Autodesk Inventor part; units mm, degrees
ref_plane "YZ Plane" through (0, 0, 0) normal (1, 0, 0) x (0, 1, 0)
ref_plane "XZ Plane" through (0, 0, 0) normal (0, 1, 0) x (-1, 0, 0)
ref_plane "XY Plane" through (0, 0, 0) normal (0, 0, 1) x (1, 0, 0)
sketch "Sketch1" plane through (0, 0, 0) normal (1, 0, 0) x (0, 1, 0)
  line L0 (0, 0) -> (10, 0)
  line L1 (10, 0) -> (10, 20)
  line L2 (10, 20) -> (5, 40)
  line L3 (5, 40) -> (0, 40)
  line L4 (0, 40) -> (0, 0)
  dimension "d0" = 10
  dimension "d1" = 5
  dimension "d2" = 20
  dimension "d3" = 20
extrude "Extrusion1" add sketch "Sketch1" along normal mid plane 20
sketch "Sketch2" plane through (-10, 0, 40) normal (0, 0, 1) x (1, 0, 0)
  line L0 (7.1, -1) -> (12.9, -1)
  line L1 (12.9, -1) -> (12.9, 0)
  line L2 (12.9, 0) -> (7.1, 0)
  line L3 (7.1, 0) -> (7.1, -1)
  line L4 (7.1, -1) -> (12.9, 0) construction
  line L5 (12.9, -1) -> (7.1, 0) construction
  line L6 (0, 0) -> (20, 0)
  point P0 (10, 0)
  point P1 (10, -0.5)
  point P2 (10, 0)
  dimension "d6" = 5.8
  dimension "d7" = 1
extrude "Extrusion2" add sketch "Sketch2" against normal up to surface (40 mm away)
sketch "Sketch5" plane through (10, 0, 0) normal (1, 0, 0) x (0, 0, -1)
  line L0 (-12.875, 11) -> (-7.125, 11)
  line L1 (-7.125, 11) -> (-7.125, 10)
  line L2 (-7.125, 10) -> (-12.875, 10)
  line L3 (-12.875, 10) -> (-12.875, 11)
  line L4 (-12.875, 11) -> (-7.125, 10) construction
  line L5 (-7.125, 11) -> (-12.875, 10) construction
  line L6 (0, 10) -> (-20, 10)
  point P0 (0, 0)
  point P1 (-10, 10.5)
  point P2 (-10, 10)
  dimension "d24" = 5.75
  dimension "d25" = 1
extrude "Extrusion3" add sketch "Sketch5" against normal up to surface (20 mm away)
chamfer "Chamfer1" distance 1 angle 45 1 edges at (0, 11, 7.125)
sketch "Sketch3" plane through (-10, 10, 20) normal (0, 1, 0) x (1, 0, 0)
  line L0 (0, -20) -> (20, -20)
  line L1 (20, 0) -> (20, -20)
  line L2 (0, 0) -> (20, 0)
  line L3 (0, -20) -> (0, 0)
  point P0 (10, 20)
  point P1 (10, -10)
  point P2 (10, 0)
  point P3 (0, -10)
hole "Hole1" at (0, 10, 30) direction (0, -1, 0) diameter 5.5 end through all counterbore diameter 10 counterbore depth 5
sketch "Sketch4" plane through (-2.9, -1, 40) normal (0, -1, 0) x (1, 0, 0)
  line L0 (-7.1, -20) -> (12.9, -20)
  line L1 (12.9, -40) -> (12.9, -32.875)
  line L2 (12.9, -40) -> (-7.1, -40)
  line L3 (-7.1, -20) -> (-7.1, -27.125)
  line L4 (-7.1, -32.875) -> (12.9, -32.875)
  line L5 (-7.1, -32.875) -> (-7.1, -40)
  line L6 (12.9, -27.125) -> (-7.1, -27.125)
  line L7 (12.9, -27.125) -> (12.9, -20)
  line L8 (-7.1, -32.875) -> (12.9, -32.875)
  line L9 (2.9, -32.875) -> (2.9, -27.125) construction
  line L10 (12.9, -27.125) -> (-7.1, -27.125)
  point P0 (2.9, -40)
  point P1 (2.9, -30)
  point P2 (-7.1, -23.5625)
  point P3 (2.9, -20)
  point P4 (2.9, -30)
hole "Hole2" at (0, -1, 10) direction (0, 1, 0) diameter 5.5 end through all counterbore diameter 10 counterbore depth 7.25
fillet "Fillet1" radius 1 5 edges at (0, 5, 40) (-10, 7.5, 30) (10, 7.5, 30) (10, 2.5, 40) (-10, 2.5, 40)
properties part number "Y-Axis_Extursion_Mount_LM3041" material "ABS Plastic"
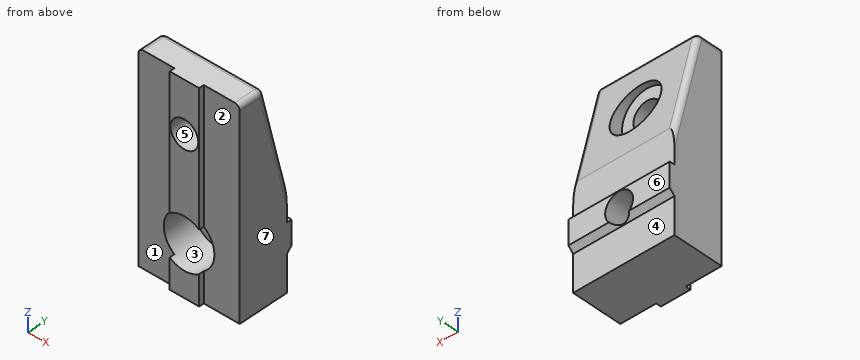
Geometry check sheet. Reference: the model listing, model coordinates, mm. Face numbers are marked on the shaded views. A direction names the side the tool comes from. Round coordinates to 2 decimals unless told otherwise and drop trailing zeros. Write each loop counter-clockwise with the first axis right and the second up, starting at its lowest first coordinate (ties: lowest second). Pieces come first, ordered by that corner, then holes. Notation, with made-up numbers: (-8, 57.25) - (46, 57.25) arc R13 ccw to (46, 79.25) - close; hole circle Ø11 at (12.25, -11). An arc over 180 degrees is marked (long way). Write each question's results on one line, items separated by ' | '.
(1) Depth check by flat-ended pin: pin 1 Ø8 at (x, z) = (0, 30) entering from +Y; pin 2 Ø5.5 at (x, z) = (-0.5, 16.5) entering from +Y; pin 3 Ø8 at (x, z) = (0, 10) entering from -Y. Enter the tip coordinate at first touch or a pass-through.
Computed:
pin 1: stops at y = 5 | pin 2: stops at y = 10 | pin 3: stops at y = 6.25
(2) Sectioned sample at B-B, the plane z = 10. Enter the section's corners in (x, y).
Computed:
outline: (-10, 0) - (-5, 0) - (-5, 6.25) - (-2.75, 6.25) - (-2.75, 11) - (-10, 11) - close; (2.75, 6.25) - (5, 6.25) - (5, 0) - (10, 0) - (10, 11) - (2.75, 11) - close
(3) Thickness scan on probe 1 along Z at (x, y) = (0, 2.25); probe 2 along X at (y, z) = (4.75, 10); probe 3 along X at (y, z) = (2.95, 30). Record the ranges inside material, lowest first. Write a range as from..to.
Computed:
probe 1: z = 0..5, 15..27.25, 32.75..40 | probe 2: x = -10..-5, 5..10 | probe 3: x = -10..-2.75, 2.75..10
(4) Sectioned sample at C-C, the plane x = 0. Count the separate pieces of the cut face and the enclosed holes in it, plus the area to 3 significant figures.
Computed:
separate pieces: 3 | enclosed holes: 0 | area: 239 mm^2
(5) Sectioned sample at A-A, the plane y = 2. Enter the section's corners in (x, z).
Computed:
outline: (-10, 0) - (10, 0) - (10, 39) arc R1 ccw to (9, 40) - (-9, 40) arc R1 ccw to (-10, 39) - close; hole circle Ø10 at (0, 10); hole circle Ø5.5 at (0, 30)
(6) Set-up check for the marked faces 1, 2, 3 and 4: record each of +Z, -Z, +X, -X, +Y, -Y from which the full face is reachable in a straight line by a thin tool's end or side.
Computed:
face 1: +Z, -Z, -X, -Y | face 2: +Z, -Z, +X, -Y | face 3: -Y | face 4: -Z, +X, -X, +Y
(7) Draft check along X on the marked faces 5, 6 and 7. Enter one of: pulls with the +X half, pulls with the -X half, needs draft (parallel to the pull), parting line crosses it, or undercut.
Computed:
face 5: undercut | face 6: needs draft | face 7: pulls with the +X half
(8) Sectioned sample at D-D, the plane z = 14.5. Enter the section's corners in (x, y).
Computed:
outline: (-10, 0) - (-2.9, 0) - (-2.9, -1) - (-2.18, -1) - (-2.18, 6.25) - (2.18, 6.25) - (2.18, -1) - (2.9, -1) - (2.9, 0) - (10, 0) - (10, 10) - (-10, 10) - close
